CAD build for the part. Positions are in the model's coordinates, mm. Face numbers are marked on the shaded views. A direction names the side the tool comes from. Coordinates: 2 decimals unless noted, no trailing zeros. Loops run counter-clockwise (first coordinate to the right, second up) from the corner with the lowest first, then second, coordinate; pieces in that order, holes last. Notation, with made-up numbers: (-33, -23.5) -> (3, -23.5) arc R16 ccw to (3, -15.5) -> close; hole circle Ø10 at (-12, 12.25). An arc over 180 degrees is marked (long way). Return JSON: item names as keys, results as strings. Group by question number.
(1) Saw through at A-A on x = 0. Write the cut outline in (y, z) (1 decimal).
(2) Saw through at C-C on y = -2. Write the cut outline in (x, z), then the cut area to 3 significant figures.
(3) Saw through at D-D on z = 3.25. Write the cut outline in (x, y), then the cut area to 3 significant figures.
(4) Tool access for the marked faces 4 and 5: list every direction of +Z, -Z, +X, -X, +Y, -Y with a clear straight run to the whole face (end or side of a thin tool).
(5) Probe L1, parallel to Y at x = 0, z = 1.65; L2, parallel to Z at x = -2.5, y = 1.25; L3, parallel to Z at x = -0.5, y = 1.75. List the from-to ranges inside material, lowest first.
(6) Flat gauge pins, fed straight in: pin 1 Ø1.5 at (x, y) = (2.5, 0.5) entering from +Z; pin 2 Ø1.5 at (y, z) = (1, 1.5) entering from -X; pin 3 Ø1.5 at (y, z) = (1, 2.5) entering from -X. Where does each tip first touch, or does it go through?
(7) Mould opens along X. For the marked faces 1, 2 and 3 say: pulls with the +X half, pulls with the -X half, needs draft (parallel to the pull), parting line crosses it, or undercut.
```python
from build123d import *

# Parameters (mm, degrees)
F0_R     = 3.175
F1_DEPTH = 1.190625
F2_R     = 2.282031
F3_DEPTH = 3.175
F4_R     = 1.5875
F5_DEPTH = 0.79375
F6_R     = 0.889
F7_DEPTH = 5.160375


with BuildPart() as f1:
    # F0 (on Top) → F1 (new body)
    with BuildSketch(Plane.XY):
        Circle(F0_R)
    extrude(amount=F1_DEPTH)

    # F2 (on face) → F3 (join)
    with BuildSketch(Plane.XY.offset(1.190625)):
        Circle(F2_R)
    extrude(amount=F3_DEPTH)

    # F4 (on face) → F5 (join)
    with BuildSketch(Plane.XY.offset(4.365625)):
        Circle(F4_R)
    extrude(amount=F5_DEPTH)

    # F6 (on face) → F7 (cut, through all)
    with BuildSketch(Plane.XY.offset(5.159375)):
        Circle(F6_R)
    extrude(amount=-F7_DEPTH, mode=Mode.SUBTRACT)


solid = f1.part
```
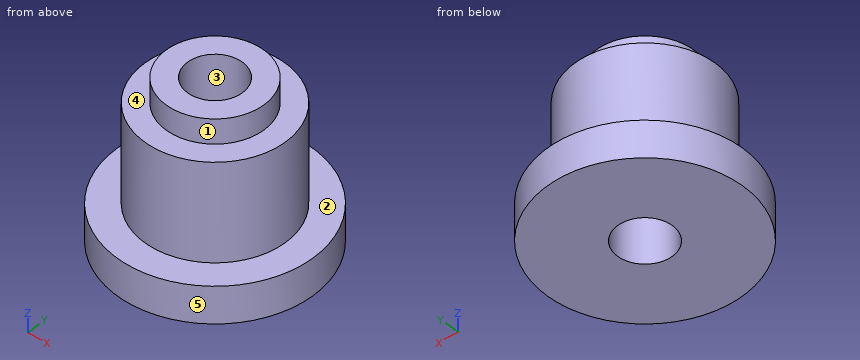
Geometry results:
{
 "1": {"outline": "(-3.2, 0) -> (-0.9, 0) -> (-0.9, 5.2) -> (-1.6, 5.2) -> (-1.6, 4.4) -> (-2.3, 4.4) -> (-2.3, 1.2) -> (-3.2, 1.2) -> close; (0.9, 0) -> (3.2, 0) -> (3.2, 1.2) -> (2.3, 1.2) -> (2.3, 4.4) -> (1.6, 4.4) -> (1.6, 5.2) -> (0.9, 5.2) -> close"},
 "2": {"outline": "(-2.47, 0) -> (2.47, 0) -> (2.47, 1.19) -> (1.1, 1.19) -> (1.1, 4.37) -> (-1.1, 4.37) -> (-1.1, 1.19) -> (-2.47, 1.19) -> close", "area": "12.9 mm²"},
 "3": {"outline": "circle Ø4.56 at (0, 0); hole circle Ø1.78 at (0, 0)", "area": "13.9 mm²"},
 "4": {"face 4": "+Z", "face 5": "+Z, -Z"},
 "5": {"L1": "-2.28 to -0.89, 0.89 to 2.28", "L2": "0 to 1.19", "L3": "0 to 4.37"},
 "6": {"pin 1": "z = 4.37", "pin 2": "x = -3.16", "pin 3": "x = -2.27"},
 "7": {"face 1": "parting line crosses it", "face 2": "needs draft", "face 3": "undercut"}
}
